Autodesk Inventor part; units mm, degrees
ref_plane "Work Plane1" through (0, 61, 0) normal (0, 1, 0) x (-1, 0, 0)
ref_plane "YZ Plane" through (0, 0, 0) normal (1, 0, 0) x (0, 1, 0)
ref_plane "XY Plane" through (0, 0, 0) normal (0, 0, 1) x (1, 0, 0)
sketch "Sketch1" plane through (0, 0, 0) normal (0, 1, 0) x (-1, 0, 0)
  circle A0 centre (7, 0) radius 5
  circle A1 centre (-7, 0) radius 5
  line L0 (7, 0) -> (-7, 0) construction
  line L1 (12, 0) -> (2, 0)
  line L2 (-2, 0) -> (-12, 0)
  circle A2 centre (-7, 0) radius 0.35
  circle A3 centre (7, 0) radius 0.35
  point P0 (0, 0)
  point P1 (0, 0)
  dimension "d0" = 10
  dimension "d1" = 14
  dimension "d8" = 0.7
sketch "Sketch2" plane through (0, 0, 0) normal (0, 0, 1) x (1, 0, 0)
  line L0 (7, 0) -> (7, 50)
  line L1 (-7, 0) -> (-7, 50)
  line L2 (-7, 0) -> (7, 0) construction
  arc A0 (7, 50) -> (-7, 50) centre (0, 50) ccw
  point P0 (0, 0)
  point P1 (0, 0)
  dimension "d2" = 14
  dimension "d3" = 50
sweep "Sweep1" add profiles "Sketch1" path "Sketch2" contours L2 A2 A1 | A1 L2 A2 | A2 L2 | L2 A2
revolve "Revolution1" add sketch "Sketch1" angle 360 about axis through (-7, 0, 0) along (1, 0, 0) picked at (3.6018, 0.4268) picked at (7.0663, 0.096) contours L1 A3 A0 | L1 A3
revolve "Revolution2" add sketch "Sketch1" angle 360 about axis through (2, 0, 0) along (1, 0, 0) picked at (-10.3982, 0.4268) picked at (-6.9337, 0.096) contours L2 A2 A1 | L2 A2
extrude "Extrusion1" add sketch "Sketch1" against normal blind 30 contours A3 L1 | L1 A3 | A2 L2 | L2 A2
ref_plane "Work Plane1" through (0, 61, 0) normal (0, 1, 0) x (-1, 0, 0)
sketch "Sketch3" plane through (0, 61, 0) normal (0, 1, 0) x (-1, 0, 0)
  circle A0 centre (0, 0) radius 1.5
  dimension "d12" = 3
extrude "Extrusion2" add sketch "Sketch3" along normal blind 4
fillet "Fillet1" radius 1.5 1 edges at (1.5, 65, 0)
properties part number "Flashbulb-DU8902" material "Phenolic Resin"
Read the model definition and answer for the solid it produces. Units are mm, in the model's axes. Give positions to 0.01 mm unless a question says otherwise; leave off trailing zeros. Order: outer loops, then holes, each group sorted by start corner. A loop starts at its lowest first (then second) coordinate and runs counter-clockwise, first axis right, second up.
(1) Given pin 1 (1.5 mm diameter, centred on x = 2, z = -1.5, fed in from -Y); pin 2 (6 mm diameter, centred on y = -14, z = -2, fed in from +X); pin 3 (1.5 mm diameter, centred on x = 5.5, y = 6, fed in from -Z), each flat-ended and moving along its own axis, determine where each tip first touches the part or whether it passes through.
(2) Find section C-C (x = 0). Give the vertices of the cut face in (y, z).
(3) For a pull along X with two mould halves and no side action, classify faces 1 (the cylindrical face through (-2.23, 24.65, 1.5)), 2 (the cylindrical face through (0.195, 62.623, -1.487)), 3 (the cylindrical face through (2.23, 25.35, 1.5)) as released by +X, released by -X, zero draft, split by the parting line, or undercut.
(4) Find section A-A (y = -12.5). Give the vertices of the cut face in (x, z), plus the area to 3 significant figures.
(5) Find section B-B (z = -4). Give the vertices of the cut face in (x, y).
(6) Find section D-D (y = 14). Give the vertices of the cut face in (x, z), plus the area to 3 significant figures.
(7) Straight lines are drawn through the part: L1, parallel to X at y = -3, z = -2.75; L2, parallel to X at y = 49.5, z = 0.25; L3, parallel to Y at x = -6.75, z = -1.25. For each, find the intervals that lie inside material, in ascending order.
Result sheet:
1. pin 1: stops at y = -2.24
1. pin 2: stops at x = 7.35
1. pin 3: stops at z = -4.94
2. outline: (61.77, -1.5) - (63.5, -1.5) arc R1.5 ccw to (63.5, 1.5) - (61.77, 1.5) arc R5 ccw (long way) to start
3. face 1: undercut
3. face 2: split by the parting line
3. face 3: undercut
4. outline: circle Ø0.7 at (-7, 0); circle Ø0.7 at (7, 0)
4. area: 0.770 mm2
5. outline: (-10, 0) arc R3 ccw to (-4, 0) - (-4, 50) arc R4 cw to (4, 50) - (4, 0) arc R3 ccw to (10, 0) - (10, 50) arc R10 ccw to (-10, 50) - close
6. outline: circle Ø10 at (-7, 0); circle Ø10 at (7, 0)
6. area: 157 mm2
7. L1: x = -9.9 to -4.1, 4.1 to 9.9
7. L2: x = -11.99 to -2.01, 2.01 to 11.99
7. L3: y = -4.83 to 59.73
